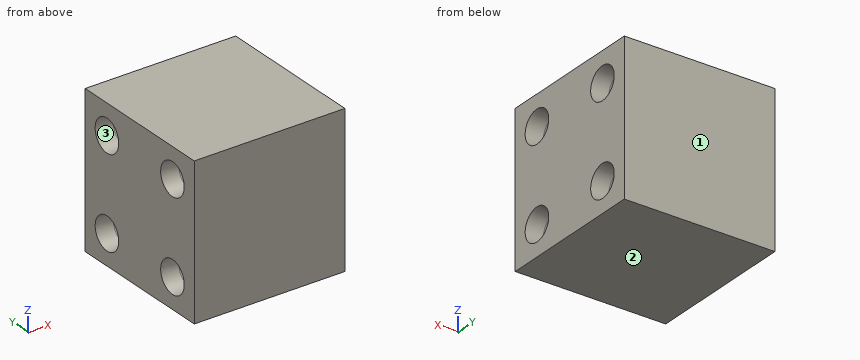
from build123d import *

# Parameters (mm, degrees)
SKETCH2_W            = 25
SKETCH2_H            = 25
BOSS_EXTRUDE1_DEPTH  = 25
LPATTERN1_COUNT      = 2
LPATTERN1_PITCH      = 15
LPATTERN1_COUNT_DIR2 = 2
LPATTERN1_PITCH_DIR2 = 15


with BuildPart() as part:
    # Sketch2 → Boss-Extrude1 (new body)
    with BuildSketch(Plane(origin=(0, 0, 0), x_dir=(1, 0, 0), z_dir=(0, 1, 0))):
        Rectangle(SKETCH2_W, SKETCH2_H)
    extrude(amount=BOSS_EXTRUDE1_DEPTH)

    # Sketch4 → CSK for M3 Oval Head Machine Screw1 (revolve, cut)
    with BuildSketch(Plane(origin=(-12.5, 20, -7.5), x_dir=(0, 0, 1), z_dir=(0, 1, 0))):
        Polygon((0, 0), (0, 11.502151548), (2.5, 10), (2.5, 2.860133251), (2.7, 0), align=None)
    csk_for_m3_oval_head_machine_screw1 = revolve(axis=Axis((-18.85, 20, -7.5), (1, 0, 0)), mode=Mode.SUBTRACT)

    # LPattern1: CSK for M3 Oval Head Machine Screw1 2 × 2
    with Locations(*[(0, -i * LPATTERN1_PITCH, j * LPATTERN1_PITCH_DIR2) for i in range(LPATTERN1_COUNT) for j in range(LPATTERN1_COUNT_DIR2) if (i, j) != (0, 0)]):
        add(csk_for_m3_oval_head_machine_screw1, mode=Mode.SUBTRACT)

    # Mirror1: CSK for M3 Oval Head Machine Screw1 across plane
    add(csk_for_m3_oval_head_machine_screw1.mirror(Plane(origin=(0, 0, 0), x_dir=(0, 0, 1), z_dir=(1, 0, 0))), mode=Mode.SUBTRACT)

    # Mirror1 copy 1 sketch → Mirror1 copy 1 (revolve, cut)
    with BuildSketch(Plane(origin=(12.5, 20, 7.5), x_dir=(0, 0, 1), z_dir=(0, 1, 0))):
        Polygon((0, 0), (0, -11.502151548), (2.5, -10), (2.5, -2.860133251), (2.7, 0), align=None)
    revolve(axis=Axis((18.85, 20, 7.5), (1, 0, 0)), mode=Mode.SUBTRACT)

    # Mirror1 copy 2 sketch → Mirror1 copy 2 (revolve, cut)
    with BuildSketch(Plane(origin=(12.5, 5, -7.5), x_dir=(0, 0, 1), z_dir=(0, 1, 0))):
        Polygon((0, 0), (0, -11.502151548), (2.5, -10), (2.5, -2.860133251), (2.7, 0), align=None)
    revolve(axis=Axis((18.85, 5, -7.5), (1, 0, 0)), mode=Mode.SUBTRACT)

    # Mirror1 copy 3 sketch → Mirror1 copy 3 (revolve, cut)
    with BuildSketch(Plane(origin=(12.5, 5, 7.5), x_dir=(0, 0, 1), z_dir=(0, 1, 0))):
        Polygon((0, 0), (0, -11.502151548), (2.5, -10), (2.5, -2.860133251), (2.7, 0), align=None)
    revolve(axis=Axis((18.85, 5, 7.5), (1, 0, 0)), mode=Mode.SUBTRACT)


solid = part.part
For this review, take the finished solid that the model builds, in its own axes (mm). Face numbers are marked on the shaded views. Round coordinates to 2 decimals unless told otherwise and drop trailing zeros. Order: outer loops, then holes, each group sorted by start corner. A loop starts at its lowest first (then second) coordinate and runs counter-clockwise, first axis right, second up. Notation, with made-up numbers: M 43,84.25 L 80,84.25 A14 ccw 80,109.25 Z; hole C 26.5,-14.5 d8. An arc over 180 degrees is marked long. Write each question's results on one line, items separated by ' | '. Start each with the question number.
1. To check wall thickness, follow L1, parallel to Y at x = 5.75, z = 7.5; L2, parallel to Z at x = -6, y = 5; L3, parallel to Z at x = 10, y = 3.25. State the ranges of each line that lie inside material, in increasing order. Write a range as [from, to].
2. Draft analysis for pull direction Y (two halves, no side actions). For the marked faces 1, 2 and 3, state which applies: pulls with the +Y half, pulls with the -Y half, needs draft (parallel to the pull), parting line crosses it, or undercut.
3. Clearance check with flat-ended pins moving along their axes: pin 1 Ø4.5 at (y, z) = (20, -7.5) entering from +X; pin 2 Ø3 at (y, z) = (20, -7.5) entering from -X. State where each tip first meets the part, or that it passes through.
4. Add section B-B (x = 10.5). State the section outline as (y, z) points.
5. Add section A-A (x = -7). State the section outline as (y, z) points, then the cut area to 3 significant figures.
Output values:
1) L1: [0, 2.5], [7.5, 17.5], [22.5, 25] | L2: [-12.5, -10], [-5, 5], [10, 12.5] | L3: [-12.5, -9.32], [-5.68, 5.68], [9.32, 12.5]
2) face 1: pulls with the +Y half | face 2: needs draft | face 3: undercut
3) pin 1: x = 2.35 | pin 2: x = -1.9
4) outline: M 0,-12.5 L 25,-12.5 L 25,12.5 L 0,12.5 Z; hole C 5,-7.5 d5.12; hole C 5,7.5 d5.12; hole C 20,-7.5 d5.12; hole C 20,7.5 d5.12
5) outline: M 0,-12.5 L 25,-12.5 L 25,12.5 L 0,12.5 Z; hole C 5,-7.5 d5; hole C 5,7.5 d5; hole C 20,-7.5 d5; hole C 20,7.5 d5 | area: 546 mm^2
